Geometry: final body of the model. Coordinates: model frame, mm. A direction names the side the tool comes from. Round coordinates to 2 decimals unless told otherwise and drop trailing zeros. Loops run counter-clockwise (first coordinate to the right, second up) from the corner with the lowest first, then second, coordinate; pieces in that order, holes last. Notation, with made-up numbers: M 38.25,29 L 45.25,29 A16 ccw 45.25,54 Z; hole C 59,61.25 d1. An arc over 180 degrees is marked long. Return JSON: item names as keys, results as strings.
from build123d import *

# Parameters (mm, degrees)
F0_R     = 1.85
F1_DEPTH = 30
F2_R     = 1.625
F3_DEPTH = 10
F5_D     = 2.5
F5_DEPTH = 13.5
F5_TIP   = 0.7510757738


with BuildPart() as f1:
    # F0 (on Top) → F1 (new body)
    with BuildSketch(Plane.XY):
        Circle(F0_R)
    extrude(amount=F1_DEPTH)

    # F2 (on face) → F3 (cut)
    with BuildSketch(Plane.XY.offset(30)):
        Circle(F2_R)
    extrude(amount=-F3_DEPTH, mode=Mode.SUBTRACT)

    # F5
    with Locations(Plane(origin=(0, 0, 0), x_dir=(1, 0, 0), z_dir=(0, 0, -1))):
        with Locations((0, 0)):
            Hole(F5_D / 2, depth=F5_DEPTH)
            with Locations((0, 0, -(F5_DEPTH + F5_TIP / 2))):  # 118° drill point
                Cone(0, F5_D / 2, F5_TIP, mode=Mode.SUBTRACT)


solid = f1.part
Q1. Material intervals for L1, parallel to Y at x = 0, z = 24.25 (3 decimals); L2, parallel to Y at x = 0, z = 4.5; L3, parallel to X at y = 0.35, z = 8.25, sorted ascending.
Determined:
{"L1": "y = -1.85 to -1.625, 1.625 to 1.85", "L2": "y = -1.85 to -1.25, 1.25 to 1.85", "L3": "x = -1.82 to -1.2, 1.2 to 1.82"}
Q2. Section query C-C (z = 28.25). Output: boundary loops of the cut face in (x, y) (3 decimals).
Determined:
{"outline": "C 0,0 d3.7; hole C 0,0 d3.25"}
Q3. Pull-direction query (X, two-part tool) for faces 1 (the cylindrical face through (-0.401, -1.806, 14.79)), 2 (the cylindrical face through (0.27, 1.22, 6.84)); classes: pulls with the +X half, pulls with the -X half, needs draft (parallel to the pull), parting line crosses it, or undercut.
Determined:
{"face 1": "parting line crosses it", "face 2": "undercut"}
Q4. Section query B-B (z = 17.5). Output: boundary loops of the cut face in (x, y).
Determined:
{"outline": "C 0,0 d3.7"}
Q5. Reachability of faces 3 (the cylindrical face through (-1.29, -0.99, 25.07)), 4 (the conical face through (-0.05, 0.21, 14.12)) from +Z, -Z, +X, -X, +Y, -Y: full face, straight path, thin tool, end or side. Return the list, or none.
Determined:
{"face 3": "+Z", "face 4": "-Z"}
Q6. Pin query (flat end, axial travel): pin 1 (1.5 mm diameter, centred on y = 1, z = 17.5, fed in from -X); pin 2 (1 mm diameter, centred on x = 0, y = 0, fed in from +Z). Return the tip coordinate at first contact, or that it passes through.
Determined:
{"pin 1": "stops at x = -1.83", "pin 2": "stops at z = 20"}
Q7. Section query A-A (z = 10.25). Output: boundary loops of the cut face in (x, y).
Determined:
{"outline": "C 0,0 d3.7; hole C 0,0 d2.5"}
